Read the model definition and answer for the solid it produces. Units are mm, in the model's axes. Face numbers are marked on the shaded views. Coordinates: 2 decimals unless noted, no trailing zeros. Loops run counter-clockwise (first coordinate to the right, second up) from the corner with the lowest first, then second, coordinate; pieces in that order, holes last. Notation, with made-up numbers: (-15, -3.75) -> (11, -3.75) arc R18 cw to (11, 20.25) -> close; hole circle Ø1 at (77, 43). An arc over 180 degrees is marked (long way). Answer as a JSON object with one key per item and string values. Group by question number.
Q1. The part is cut by section D-D on x = 6. Write down the section's boundary in (y, z).
Q2. Determine the mould class of the marked faces 1, 2, 3 and 4 for opening direction X: released by +X, released by -X, zero draft, split by the parting line, or undercut.
Q3. Straight lines are drawn through the part: line 1 along X through (y, z) = (17.25, 15); line 2 along X through (y, z) = (11.25, 0); line 3 along Z through (x, y) = (11, 10). For each, find the intervals that lie inside material, in ascending order. Write a range as [from, to].
Q4. Each of these flat-tipped pins is pushed along its axis until it touches: P1, Ø5, axis at y = 13, z = -11.5, coming from the -X side; P2, Ø1.8, axis at y = 11, z = 12, coming from the +X side; P3, Ø2, axis at y = 8.5, z = -1.5, coming from the +X side; P4, Ø5, axis at x = 5, y = 9.5, coming from the -Z side. Where does it stop, or does it pass through?
Q5. The part is cut by section B-B on z = -4. Write down the section's boundary in (x, y).
Q6. The part is cut by section C-C on y = 5. Write down the section's boundary in (x, z), and give its area (3 significant figures).
Q7. The part is cut by section A-A on x = -10.5. Write down the section's boundary in (y, z).
Autodesk Inventor part; units mm, degrees
ref_plane "YZ Plane" through (0, 0, 0) normal (1, 0, 0) x (0, 1, 0)
ref_plane "XZ Plane" through (0, 0, 0) normal (0, 1, 0) x (-1, 0, 0)
ref_plane "XY Plane" through (0, 0, 0) normal (0, 0, 1) x (1, 0, 0)
sketch "Sketch1" plane through (0, 0, 0) normal (0, 1, 0) x (-1, 0, 0)
  arc A0 (-1, 13.4629) -> (1, 13.4629) centre (0, 0) ccw
  arc A1 (-17, 0) -> (17, 0) centre (0, 0) ccw
  line L0 (17, 0) -> (17, 19.8)
  line L1 (-17, 19.8) -> (-17, 0)
  line L2 (-1, 19.8) -> (-1, 13.4629)
  line L3 (1, 19.8) -> (1, 13.4629)
  line L4 (17, 19.8) -> (1, 19.8)
  line L5 (-1, 19.8) -> (-17, 19.8)
  dimension "d0" = 27
  dimension "d1" = 34
extrude "Extrusion1" add sketch "Sketch1" along normal blind 20
sketch "Sketch2" plane through (17, 0, 19.8) normal (1, 0, 0) x (0, 0, -1)
  line L0 (0, 0) -> (0, 20)
  line L1 (3.52, 13) -> (9.52, 13)
  line L2 (9.52, 13) -> (9.52, 7)
  line L3 (9.52, 7) -> (3.52, 7)
  line L4 (3.52, 7) -> (3.52, 13)
  line L5 (3.52, 13) -> (9.52, 7) construction
  line L6 (9.52, 13) -> (3.52, 7) construction
  point P0 (6.52, 10)
  dimension "d7" = 6.52
  dimension "d15" = 6
  dimension "d16" = 6
hole "Hole1" at (17, 10, 13.28) direction (-1, 0, 0) diameter 5.791 end through all
extrude "Extrusion2" cut sketch "Sketch2" against normal blind 3.3
properties part number "slik_clamp_head38_collar"
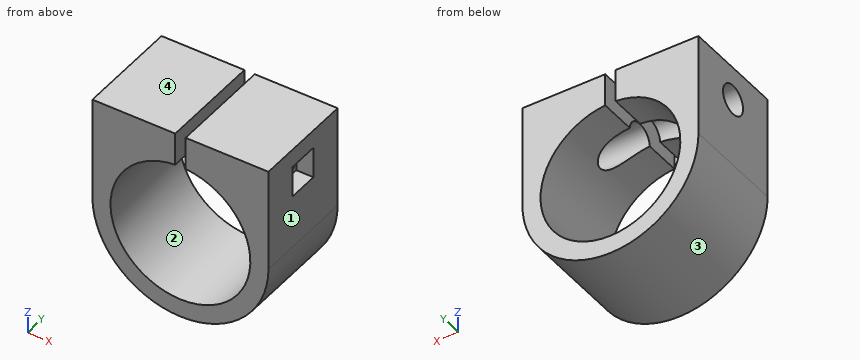
Final values:
{
 "1": {"outline": "(0, -15.91) -> (20, -15.91) -> (20, -12.09) -> (0, -12.09) -> close; (0, 12.09) -> (7.36, 12.09) arc R2.9 cw (long way) to (12.64, 12.09) -> (20, 12.09) -> (20, 19.8) -> (0, 19.8) -> close"},
 "2": {"face 1": "released by +X", "face 2": "undercut", "face 3": "split by the parting line", "face 4": "zero draft"},
 "3": {"line 1": "x = [-17, -1], [1, 17]", "line 2": "x = [-17, -13.5], [13.5, 17]", "line 3": "z = [-12.96, -7.83], [7.83, 10.38], [16.18, 19.8]"},
 "4": {"P1": "stops at x = -14.42", "P2": "passes through", "P3": "stops at x = 16.99", "P4": "stops at z = -16.82"},
 "5": {"outline": "(-16.52, 0) -> (-12.89, 0) -> (-12.89, 20) -> (-16.52, 20) -> close; (12.89, 0) -> (16.52, 0) -> (16.52, 20) -> (12.89, 20) -> close"},
 "6": {"outline": "(-17, 0) arc R17 ccw to (17, 0) -> (17, 19.8) -> (1, 19.8) -> (1, 13.46) arc R13.5 cw (long way) to (-1, 13.46) -> (-1, 19.8) -> (-17, 19.8) -> close", "area": "542 mm2"},
 "7": {"outline": "(0, -13.37) -> (20, -13.37) -> (20, -8.49) -> (0, -8.49) -> close; (0, 8.49) -> (20, 8.49) -> (20, 19.8) -> (0, 19.8) -> close; hole circle Ø5.79 at (10, 13.28)"}
}
